```python
from build123d import *

# Parameters (mm, degrees)
SKETCH1_W                                           = 220
SKETCH1_H                                           = 55
BOSS_EXTRUDE1_DEPTH                                 = 17.5
SKETCH2_W                                           = 80
SKETCH2_H                                           = 47
CUT_EXTRUDE1_DEPTH                                  = 5
CBORE_FOR_M5_HEX_SOCKET_HEAD_CAP_SCREW1_D           = 5.5
CBORE_FOR_M5_HEX_SOCKET_HEAD_CAP_SCREW1_CBORE_D     = 10
CBORE_FOR_M5_HEX_SOCKET_HEAD_CAP_SCREW1_CBORE_DEPTH = 24
SKETCH10_W                                          = 18
SKETCH10_H                                          = 12
CUT_EXTRUDE4_DEPTH                                  = 223.401663663
SKETCH5_W                                           = 100
SKETCH5_H                                           = 80
CUT_EXTRUDE2_DEPTH                                  = 119.664442863
SKETCH6_W                                           = 22
SKETCH6_H                                           = 44.180340856
CUT_EXTRUDE3_DEPTH                                  = 119.664442863
FILLET1_R                                           = 5
M5_TAPPED_HOLE1_D                                   = 4.2
M5_TAPPED_HOLE1_DEPTH                               = 14
M5_TAPPED_HOLE1_TIP                                 = 1.2618073
M6_TAPPED_HOLE1_D                                   = 5
M6_TAPPED_HOLE1_DEPTH                               = 35
M6_TAPPED_HOLE1_TIP                                 = 1.502151548
F_6_0MM_DOWEL_HOLE1_D                               = 6
F_6_0MM_DOWEL_HOLE1_DEPTH                           = 20
F_6_0MM_DOWEL_HOLE1_TIP                             = 1.802581857


with BuildPart() as part:
    # Sketch1 → Boss-Extrude1 (new, symmetric)
    with BuildSketch(Plane(origin=(0, 0, 0), x_dir=(1, 0, 0), z_dir=(0, 1, 0))):
        Rectangle(SKETCH1_W, SKETCH1_H)
    extrude(amount=BOSS_EXTRUDE1_DEPTH, both=True)

    # Sketch2 → Cut-Extrude1 (cut)
    with BuildSketch(Plane(origin=(0, 17.5, 0), x_dir=(1, 0, 0), z_dir=(0, 1, 0))):
        with Locations((-75, 1)):
            Rectangle(SKETCH2_W, SKETCH2_H)
    cut_extrude1 = extrude(amount=-CUT_EXTRUDE1_DEPTH, mode=Mode.SUBTRACT)

    # Mirror1: Cut-Extrude1 across plane
    add(cut_extrude1.mirror(Plane(origin=(0, 0, 0), x_dir=(0, 0, 1), z_dir=(1, 0, 0))), mode=Mode.SUBTRACT)

    # CBORE for M5 Hex Socket Head Cap Screw1 (through all)
    with Locations(Plane(origin=(0, -17.5, 0), x_dir=(-1, 0, 0), z_dir=(0, -1, 0))):
        with Locations((-100, 20), (-70, 20), (-70, -18), (-100, -18), (70, 20), (100, 20), (100, -18), (70, -18)):
            CounterBoreHole(CBORE_FOR_M5_HEX_SOCKET_HEAD_CAP_SCREW1_D / 2, CBORE_FOR_M5_HEX_SOCKET_HEAD_CAP_SCREW1_CBORE_D / 2, CBORE_FOR_M5_HEX_SOCKET_HEAD_CAP_SCREW1_CBORE_DEPTH)

    # Sketch10 → Cut-Extrude4 (cut, through all)
    with BuildSketch(Plane.ZY.offset(110)):
        with Locations((18.5, -11.5)):
            Rectangle(SKETCH10_W, SKETCH10_H)
    extrude(amount=-CUT_EXTRUDE4_DEPTH, mode=Mode.SUBTRACT)

    # Sketch5 → Cut-Extrude2 (cut, through all)
    with BuildSketch(Plane.XZ.offset(17.5)):
        with Locations((0, -52.5)):
            Rectangle(SKETCH5_W, SKETCH5_H)
    extrude(amount=-CUT_EXTRUDE2_DEPTH, mode=Mode.SUBTRACT)

    # Sketch6 → Cut-Extrude3 (cut, through all)
    with BuildSketch(Plane.XZ.offset(17.5)):
        with Locations((0, 31.590170428)):
            Rectangle(SKETCH6_W, SKETCH6_H)
    extrude(amount=-CUT_EXTRUDE3_DEPTH, mode=Mode.SUBTRACT)

    # Fillet1
    fillet1_edges = [part.edges().sort_by_distance(p)[0] for p in [
        (-35, 15, 22.5),
        (35, 15, 22.5),
    ]]
    fillet(fillet1_edges, radius=FILLET1_R)

    # M5 Tapped Hole1
    with Locations(Plane(origin=(0, 0, -12.5), x_dir=(-1, 0, 0), z_dir=(0, 0, -1))):
        with Locations((-17, 12), (17, 12), (17, -12), (-17, -12)):
            Hole(M5_TAPPED_HOLE1_D / 2, depth=M5_TAPPED_HOLE1_DEPTH)
            with Locations((0, 0, -(M5_TAPPED_HOLE1_DEPTH + M5_TAPPED_HOLE1_TIP / 2))):  # 118° drill point
                Cone(0, M5_TAPPED_HOLE1_D / 2, M5_TAPPED_HOLE1_TIP, mode=Mode.SUBTRACT)

    # M6 Tapped Hole1
    with Locations(Plane(origin=(0, -17.5, 0), x_dir=(-1, 0, 0), z_dir=(0, -1, 0))):
        with Locations((-101.5, 0.5), (-81.5, 10.5), (-61.5, 0.5)):
            Hole(M6_TAPPED_HOLE1_D / 2, depth=M6_TAPPED_HOLE1_DEPTH)
            with Locations((0, 0, -(M6_TAPPED_HOLE1_DEPTH + M6_TAPPED_HOLE1_TIP / 2))):  # 118° drill point
                Cone(0, M6_TAPPED_HOLE1_D / 2, M6_TAPPED_HOLE1_TIP, mode=Mode.SUBTRACT)

    # Ø6.0mm Dowel Hole1
    with Locations(Plane(origin=(0, -17.5, 0), x_dir=(-1, 0, 0), z_dir=(0, -1, 0))):
        with Locations((-101.5, 10.5), (-61.5, 10.5)):
            Hole(F_6_0MM_DOWEL_HOLE1_D / 2, depth=F_6_0MM_DOWEL_HOLE1_DEPTH)
            with Locations((0, 0, -(F_6_0MM_DOWEL_HOLE1_DEPTH + F_6_0MM_DOWEL_HOLE1_TIP / 2))):  # 118° drill point
                Cone(0, F_6_0MM_DOWEL_HOLE1_D / 2, F_6_0MM_DOWEL_HOLE1_TIP, mode=Mode.SUBTRACT)


solid = part.part
```
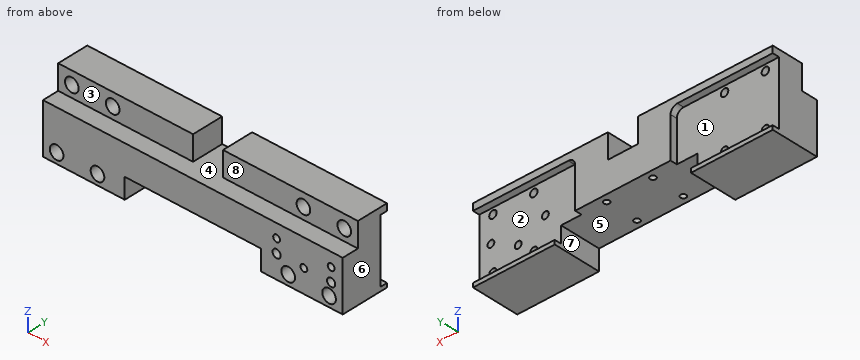
Here's how the part is built. I have some questions about the finished solid (model axes, mm). Face numbers are marked on the shaded views. A direction names the side the tool comes from. Round coordinates to 2 decimals unless told otherwise and drop trailing zeros. Loops run counter-clockwise (first coordinate to the right, second up) from the corner with the lowest first, then second, coordinate; pieces in that order, holes last. Notation, with made-up numbers: (-32.5, -36.75) -> (-12.5, -36.75) arc R7 cw to (-12.5, -29.75) -> close; hole circle Ø3 at (-2.5, -31). An arc over 180 degrees is marked (long way). Answer as CSV lines item,"result". Start each with the question number.
1. For the marked faces 1, 2, 3, 4 and 5, which set-ups out of +Z, -Z, +X, -X, +Y, -Y let a thin tool reach every point of the face, with its end or its side?
2. I need wall thicknesses on probe 1 along Y at (x, z) = (17, -2); probe 2 along X at (y, z) = (-1, 18); probe 3 along Z at (x, y) = (70, 9.6). Which ranges of each line are inside material? Lowest first, please. Write a range as from..to.
3. Imagine slicing it at C-C on x = -100. Write out the boundary of the cut face in (y, z).
4. If we mould it in two halves opening along X, with no side actions, what happens to the marked faces 6, 7 and 8? For each: pulls with the +X half, pulls with the -X half, needs draft (parallel to the pull), parting line crosses it, or undercut.
5. I'm going to push flat-ended pins straight in: P1, Ø12, axis at x = 57, z = 0.5, coming from the +Y side; P2, Ø6.5, axis at x = 70, z = -20, coming from the -Y side; P3, Ø5.5, axis at x = 17, y = 12, coming from the -Z side. Where does each tip first touch, or does it pass through?
6. Imagine slicing it at D-D on x = 54.5. Write out the boundary of the cut face in (y, z).
7. Imagine slicing it at B-B on y = 0. State how many separate pieces and enclosed holes the cut face has, plus the area to 3 significant figures.
8. Imagine slicing it at A-A on z = -0.5. Write out the boundary of the cut face in (x, y), plus the area to 3 significant figures.
Solution:
1,face 1,"-X, +Y"
1,face 2,"+X, +Y"
1,face 3,"+Z, +X, -X, -Y"
1,face 4,"+Z, -Y"
1,face 5,"-Z, +Y, -Y"
2,probe 1,"-17.5..-14.1, -9.9..9.9, 14.1..17.5"
2,probe 2,"-110..-105, -95..-75, -65..-11, 11..65, 75..95, 105..110"
2,probe 3,"-27.5..-22.75, -17.25..15.25, 20.75..27.5"
3,outline,"(-17.5, -27.5) -> (17.5, -27.5) -> (17.5, -24.5) -> (12.5, -24.5) -> (12.5, -22.75) -> (6.5, -22.75) -> (6.5, -25) -> (-17.5, -25) -> close; (-17.5, -15) -> (6.5, -15) -> (6.5, -17.25) -> (12.5, -17.25) -> (12.5, 15.25) -> (6.5, 15.25) -> (6.5, 13) -> (-5.5, 13) -> (-5.5, 9.5) -> (-17.5, 9.5) -> close; (-5.5, 23) -> (6.5, 23) -> (6.5, 20.75) -> (12.5, 20.75) -> (12.5, 22.5) -> (17.5, 22.5) -> (17.5, 27.5) -> (-5.5, 27.5) -> close"
4,face 6,"pulls with the +X half"
4,face 7,"undercut"
4,face 8,"needs draft"
5,P1,"y = 12.5"
5,P2,"y = 6.5"
5,P3,"z = -12.5"
6,outline,"(-17.5, -27.5) -> (17.5, -27.5) -> (17.5, -24.5) -> (12.5, -24.5) -> (12.5, 22.5) -> (17.5, 22.5) -> (17.5, 27.5) -> (-5.5, 27.5) -> (-5.5, 9.5) -> (-17.5, 9.5) -> close"
7,separate pieces,"1"
7,enclosed holes,"13"
7,area,"9,460 mm²"
8,outline,"(-110, -17.5) -> (59, -17.5) -> (59, 12.5) -> (35, 12.5) -> (35, 17.5) -> (-35, 17.5) -> (-35, 12.5) -> (-110, 12.5) -> close; (64, -17.5) -> (99, -17.5) -> (99, 12.5) -> (64, 12.5) -> close; (104, -17.5) -> (110, -17.5) -> (110, 12.5) -> (104, 12.5) -> close; hole circle Ø4.2 at (-17, -12); hole circle Ø4.2 at (-17, 12); hole circle Ø4.2 at (17, -12); hole circle Ø4.2 at (17, 12)"
8,area,"6,590 mm²"
